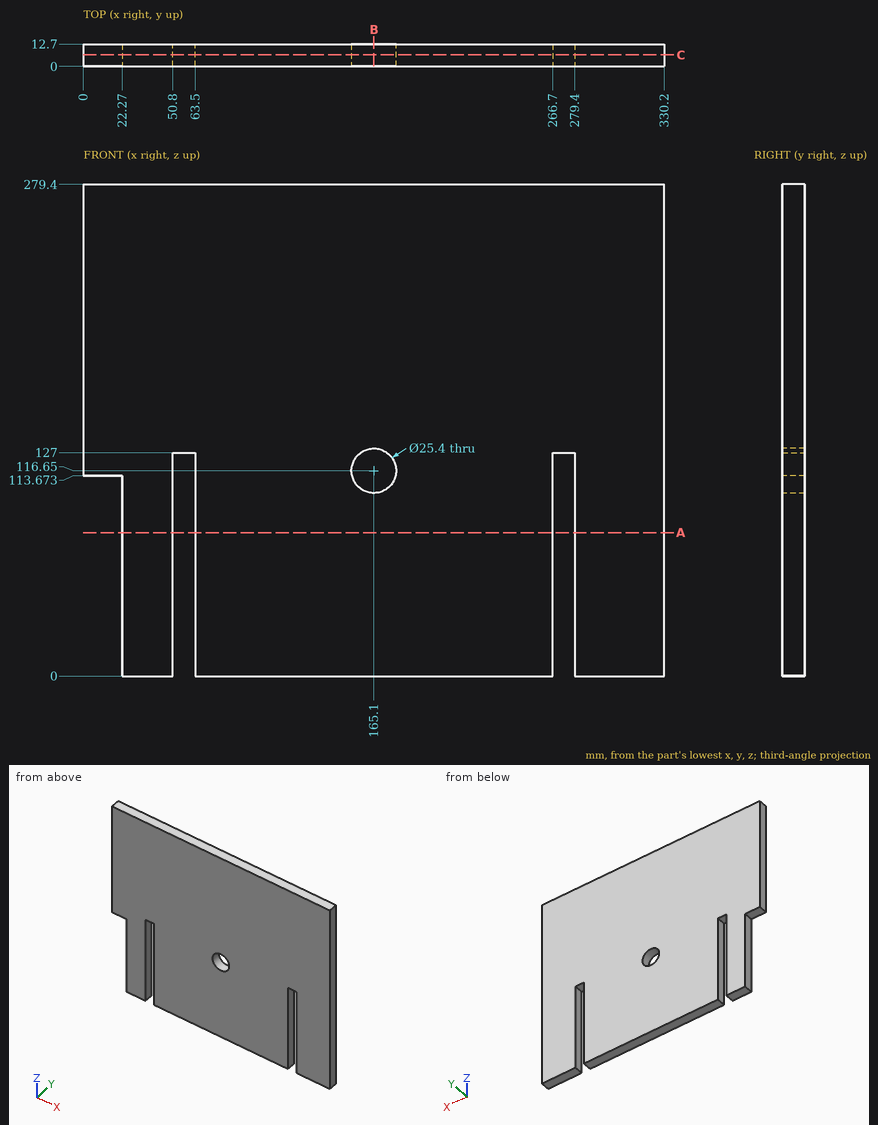
The figure shows three views and two pictorial views of one solid part (mm, origin at its lowest corner). Answer the questions. Coordinates: 2 decimals unless noted, no trailing zeros. Loops run counter-clockwise (first coordinate to the right, second up) from the corner with the lowest first, then second, coordinate; pieces in that order, holes last. Notation, with made-up numbers: (77, 59.5) -> (103, 59.5) arc R15 cw to (103, 78.5) -> close; hole circle Ø11 at (-12.5, 26). An arc over 180 degrees is marked (long way). Write item = value, one per line. Start each with the question number.
1) Straight lines are drawn through the part: line 1 (X direction, y = 5.75, z = 53); line 2 (X direction, y = 8.5, z = 116.65); line 3 (Z direction, x = 165.1, y = 7.75). For each, find the intervals that lie inside material, in ascending order. Write a range as from..to.
2) A cutting plane is placed at B-B (x = 165.1). Give the vertices of the cut face in (y, z), then the cut area to 3 significant figures.
3) Given pin 1 Ø4 at (y, z) = (4, 187) entering from -X; pin 2 Ø4 at (x, y) = (15, 4.5) entering from -Z; pin 3 Ø6.5 at (y, z) = (4, 72.5) entering from -X; pin 4 Ø4 at (x, y) = (273.5, 5) entering from -Z, each flat-ended and moving along its own axis, determine where each tip first touches the part or whether it passes through.
4) A cutting plane is placed at A-A (z = 81.5). Give the vertices of the cut face in (x, y).
5) A cutting plane is placed at C-C (y = 6.5). Give the vertices of the cut face in (x, z), then the cut area to 3 significant figures.
Responses:
q1.line_1 = 22.27..50.8, 63.5..266.7, 279.4..330.2
q1.line_2 = 0..50.8, 63.5..152.4, 177.8..266.7, 279.4..330.2
q1.line_3 = 0..103.95, 129.35..279.4
q2.outline = (0, 0) -> (12.7, 0) -> (12.7, 103.95) -> (0, 103.95) -> close; (0, 129.35) -> (12.7, 129.35) -> (12.7, 279.4) -> (0, 279.4) -> close
q2.area = 3,230 mm²
q3.pin_1 = 0
q3.pin_2 = 113.67
q3.pin_3 = 22.27
q3.pin_4 = 127
q4.outline = (22.27, 0) -> (50.8, 0) -> (50.8, 12.7) -> (22.27, 12.7) -> close; (63.5, 0) -> (266.7, 0) -> (266.7, 12.7) -> (63.5, 12.7) -> close; (279.4, 0) -> (330.2, 0) -> (330.2, 12.7) -> (279.4, 12.7) -> close
q5.outline = (0, 113.67) -> (22.27, 113.67) -> (22.27, 0) -> (50.8, 0) -> (50.8, 127) -> (63.5, 127) -> (63.5, 0) -> (266.7, 0) -> (266.7, 127) -> (279.4, 127) -> (279.4, 0) -> (330.2, 0) -> (330.2, 279.4) -> (0, 279.4) -> close; hole circle Ø25.4 at (165.1, 116.65)
q5.area = 86,000 mm²
